```python
from build123d import *

# Parameters (mm, degrees)
BOSS_EXTRUDE1_DEPTH        = 150
M2_5_START                 = -133.151532693
M2_5_CLEARANCE_SLOT1_DEPTH = 3.368059081
CIRPATTERN1_COUNT          = 4
CIRPATTERN1_ANGLE          = 62.5


# Read off the part's stored shape, not the designer's step: M2.5 Clearance Slot1
with BuildPart() as part:
    # Sketch1 → Boss-Extrude1 (new body)
    with BuildSketch(Plane(origin=(0, 0, 0), x_dir=(1, 0, 0), z_dir=(0, 1, 0))):
        with BuildLine():
            Line((-130, 0), (-133.175, 0))
            ThreePointArc((-133.175, 0), (-110.407078725, 74.47051492), (-49.888233078, 123.477709832))
            Line((-49.888233078, 123.477709832), (-48.698857144, 120.533901094))
            ThreePointArc((-48.698857144, 120.533901094), (-107.774884432, 72.695077451), (-130, 0))
        make_face()
    extrude(amount=BOSS_EXTRUDE1_DEPTH)

    # M2.5 Clearance Slot1 outline → M2.5 Clearance Slot1 (cut)
    with BuildSketch(Plane.YZ.offset(M2_5_START)):
        with BuildLine():
            ThreePointArc((1.825, -6.15), (3.175, -7.5), (4.525, -6.15))
            Line((4.525, -6.15), (4.525, -3.85))
            ThreePointArc((4.525, -3.85), (3.175, -2.5), (1.825, -3.85))
            Line((1.825, -3.85), (1.825, -6.15))
        make_face()
    m2_5_clearance_slot1 = extrude(amount=M2_5_CLEARANCE_SLOT1_DEPTH, mode=Mode.SUBTRACT)

    # CirPattern1: M2.5 Clearance Slot1 ×4 about axis
    cirpattern1_axis = Axis((0, 150, 0), (0, -1, 0))
    for i in range(1, CIRPATTERN1_COUNT):
        add(m2_5_clearance_slot1.rotate(cirpattern1_axis, i * CIRPATTERN1_ANGLE / (CIRPATTERN1_COUNT - 1)), mode=Mode.SUBTRACT)


solid = part.part
```
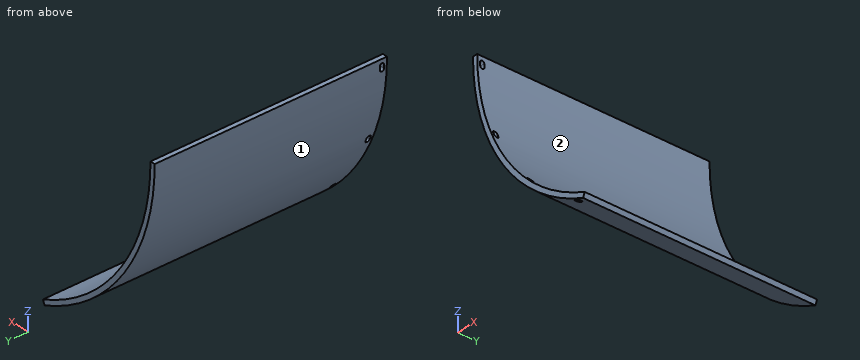
Part model, mm, in its own coordinate system. Face numbers are marked on the shaded views. Give positions to 0.01 mm unless a question says otherwise; leave off trailing zeros. Order: outer loops, then holes, each group sorted by start corner. A loop starts at its lowest first (then second) coordinate and runs counter-clockwise, first axis right, second up. Notation, with made-up numbers: M 88.5,-16 L 133.5,-16 A18 ccw 133.5,-4 Z; hole C 46,33 d5. An arc over 180 degrees is marked long. Use a Markdown table: item, result. Add a question column.
(1) Saw through at A-A, the plane y = 29.5. Give the cut face in (x, z) (3 decimals).
(2) Probe line 1 along X through (y, z) = (67.5, -24.5); line 2 along X through (y, z) = (51, -5.5); line 3 along Z through (x, y) = (-57, 117). List the from-to ranges inside material, lowest first. Write a range as [from, to].
(3) Mould opens along X. For the marked faces 1 and 2 say: +X half, -X half, draft (parallel to the pull), parting line (faces both ways), or undercut.
(4) Drop flat-ended pins along their axis: P1, Ø12, axis at x = -119.5, z = -75.5, coming from the -Y side; P2, Ø12, axis at x = -82, y = 73.5, coming from the -Z side; P3, Ø6, axis at y = 83.5, z = -86, coming from the +X side; P4, Ø5, axis at x = -84, y = 75, coming from the -Z side. Give the stop position or say it passes through.
Answer key:
| question | item | result |
|---|---|---|
| 1 | outline | M -133.175,0 A133.175 ccw -49.888,-123.478 L -48.699,-120.534 A130 cw -130,0 Z |
| 2 | line 1 | [-130.9, -127.67] |
| 2 | line 2 | [-133.06, -129.88] |
| 2 | line 3 | [-120.36, -116.84] |
| 3 | face 1 | -X half |
| 3 | face 2 | +X half |
| 4 | P1 | through |
| 4 | P2 | z = -109.36 |
| 4 | P3 | x = -94.76 |
| 4 | P4 | z = -105.32 |
